from build123d import *

# Parameters (mm, degrees)
SKETCH1_W           = 165.1
SKETCH1_H           = 63.5
BOSS_EXTRUDE1_DEPTH = 3
CUT_EXTRUDE1_REACH  = 90.496
SKETCH2_R           = 1.5


with BuildPart() as part:
    # Sketch1 → Boss-Extrude1 (new body)
    with BuildSketch(Plane(origin=(0, 0, 0), x_dir=(1, 0, 0), z_dir=(0, 1, 0))):
        Rectangle(SKETCH1_W, SKETCH1_H)
    extrude(amount=BOSS_EXTRUDE1_DEPTH)

    # Sketch2 → Cut-Extrude1 (cut, up to next)
    with BuildSketch(Plane(origin=(0, 3, 0), x_dir=(1, 0, 0), z_dir=(0, 1, 0)), mode=Mode.PRIVATE) as cut_extrude1_sk1:
        with Locations(Location((-77.47, 26.67, 0), (0, 0, 270))):
            Circle(SKETCH2_R)
    cut_extrude1_tool1 = extrude(cut_extrude1_sk1.sketch, amount=-CUT_EXTRUDE1_REACH, mode=Mode.PRIVATE) & part.part
    # Sketch2 → Cut-Extrude1 (cut, up to next)
    with BuildSketch(Plane(origin=(0, 3, 0), x_dir=(1, 0, 0), z_dir=(0, 1, 0)), mode=Mode.PRIVATE) as cut_extrude1_sk2:
        with Locations(Location((-77.47, -26.67, 0), (0, 0, 270))):
            Circle(SKETCH2_R)
    cut_extrude1_tool2 = extrude(cut_extrude1_sk2.sketch, amount=-CUT_EXTRUDE1_REACH, mode=Mode.PRIVATE) & part.part
    # Sketch2 → Cut-Extrude1 (cut, up to next)
    with BuildSketch(Plane(origin=(0, 3, 0), x_dir=(1, 0, 0), z_dir=(0, 1, 0)), mode=Mode.PRIVATE) as cut_extrude1_sk3:
        with Locations(Location((77.47, 26.67, 0), (0, 0, 270))):
            Circle(SKETCH2_R)
    cut_extrude1_tool3 = extrude(cut_extrude1_sk3.sketch, amount=-CUT_EXTRUDE1_REACH, mode=Mode.PRIVATE) & part.part
    # Sketch2 → Cut-Extrude1 (cut, up to next)
    with BuildSketch(Plane(origin=(0, 3, 0), x_dir=(1, 0, 0), z_dir=(0, 1, 0)), mode=Mode.PRIVATE) as cut_extrude1_sk4:
        with Locations(Location((77.47, -26.67, 0), (0, 0, 270))):
            Circle(SKETCH2_R)
    cut_extrude1_tool4 = extrude(cut_extrude1_sk4.sketch, amount=-CUT_EXTRUDE1_REACH, mode=Mode.PRIVATE) & part.part
    add(cut_extrude1_tool1.solids().sort_by_distance((-77.47, 3, -26.67))[0], mode=Mode.SUBTRACT)
    add(cut_extrude1_tool2.solids().sort_by_distance((-77.47, 3, 26.67))[0], mode=Mode.SUBTRACT)
    add(cut_extrude1_tool3.solids().sort_by_distance((77.47, 3, -26.67))[0], mode=Mode.SUBTRACT)
    add(cut_extrude1_tool4.solids().sort_by_distance((77.47, 3, 26.67))[0], mode=Mode.SUBTRACT)


solid = part.part
Check sheet for the modelled part. Datum: model origin and axes. Units: mm. Give positions to 0.01 mm unless a question says otherwise; leave off trailing zeros. Write each loop counter-clockwise with the first axis right and the second up, starting at its lowest first coordinate (ties: lowest second). Pieces come first, ordered by that corner, then holes. Notation, with made-up numbers: (10, 89.5) -> (68, 89.5) arc R15 cw to (68, 96.5) -> close; hole circle Ø3 at (32.5, -22.75). An arc over 180 degrees is marked (long way). One line per item, written item: value. Start each with the question number.
Item 1: Section check A-A on x = -77.47. Record the cut outline in (y, z), then the cut area to 4 significant figures.
Item 2: Draft check along Z on faces 1 (the flat face through (-1, 1, -31.75)), 2 (the flat face through (-82.55, 1, 0)), 3 (the cylindrical face through (-75.983, 1.521, -26.865)). Enter one of: +Z half, -Z half, draft (parallel to the pull), parting line (faces both ways), or undercut.
Item 3: Gauge pin test, flat ends, axial feed: pin 1 (2.5 mm diameter, centred on x = -77.47, z = -26.67, fed in from +Y); pin 2 (3.5 mm diameter, centred on x = 77.47, z = -26.67, fed in from +Y). Record the tip position at first contact, or that the pin passes through.
Item 4: Material ranges on probe 1 along Z at (x, y) = (77.47, 1.5); probe 2 along X at (y, z) = (1.75, 26.67), recorded low to high. Write a range as from..to.
Item 5: Section check B-B on z = 26.67. Record the cut outline in (x, y).
Results list:
1. outline: (0, -31.75) -> (3, -31.75) -> (3, -28.17) -> (0, -28.17) -> close; (0, -25.17) -> (3, -25.17) -> (3, 25.17) -> (0, 25.17) -> close; (0, 28.17) -> (3, 28.17) -> (3, 31.75) -> (0, 31.75) -> close
1. area: 172.5 mm²
2. face 1: -Z half
2. face 2: draft
2. face 3: undercut
3. pin 1: through
3. pin 2: y = 3
4. probe 1: -31.75..-28.17, -25.17..25.17, 28.17..31.75
4. probe 2: -82.55..-78.97, -75.97..75.97, 78.97..82.55
5. outline: (-82.55, 0) -> (-78.97, 0) -> (-78.97, 3) -> (-82.55, 3) -> close; (-75.97, 0) -> (75.97, 0) -> (75.97, 3) -> (-75.97, 3) -> close; (78.97, 0) -> (82.55, 0) -> (82.55, 3) -> (78.97, 3) -> close
